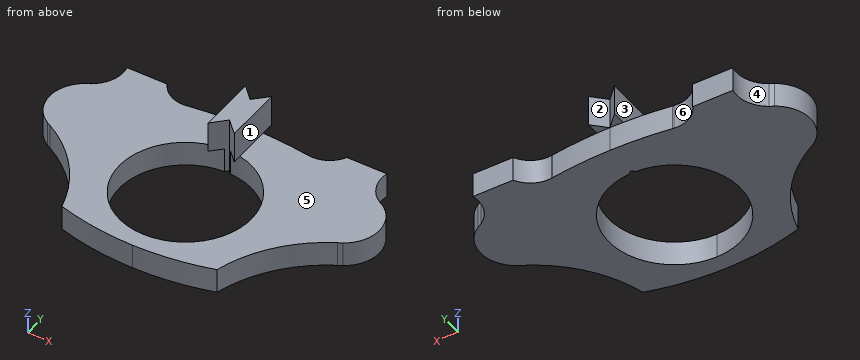
from build123d import *

# Parameters (mm, degrees)
F1_DEPTH = 8
F3_DEPTH = 10
F5_DEPTH = 25


with BuildPart() as f1:
    # F0 (on Top) → F1 (new body)
    with BuildSketch(Plane.XY):
        with BuildLine():
            Line((42.068422, 21.54067), (29.081911, 21.54067))
            ThreePointArc((29.081911, 21.54067), (25.256656, 17.577108), (19.841552, 16.567634))
            ThreePointArc((19.841552, 16.567634), (19.64703, 16.594249), (19.453131, 16.62508))
            ThreePointArc((19.453131, 16.62508), (9.752315, 17.686936), (0, 18.041513))
            ThreePointArc((0, 18.041513), (-9.752315, 17.686936), (-19.453131, 16.62508))
            ThreePointArc((-19.453131, 16.62508), (-19.64703, 16.594249), (-19.841552, 16.567634))
            ThreePointArc((-19.841552, 16.567634), (-25.256656, 17.577108), (-29.081911, 21.54067))
            Line((-29.081911, 21.54067), (-42.068422, 21.54067))
            ThreePointArc((-42.068422, 21.54067), (-42.606666, 15.286638), (-46.635796, 10.473247))
            ThreePointArc((-46.635796, 10.473247), (-47.308086, 10.078485), (-48.007976, 9.735025))
            ThreePointArc((-48.007976, 9.735025), (-53.385548, -0.095187), (-47.845987, -9.835033))
            ThreePointArc((-47.845987, -9.835033), (-47.228549, -10.153727), (-46.616208, -10.482108))
            ThreePointArc((-46.616208, -10.482108), (-33.037563, -21.996435), (-25.116532, -37.940607))
            ThreePointArc((-25.116532, -37.940607), (-12.686785, -40.637885), (0, -41.543091))
            ThreePointArc((0, -41.543091), (12.686785, -40.637885), (25.116532, -37.940607))
            ThreePointArc((25.116532, -37.940607), (33.037563, -21.996435), (46.616208, -10.482108))
            ThreePointArc((46.616208, -10.482108), (47.228549, -10.153727), (47.845987, -9.835033))
            ThreePointArc((47.845987, -9.835033), (53.385548, -0.095187), (48.007976, 9.735025))
            ThreePointArc((48.007976, 9.735025), (47.308086, 10.078485), (46.635796, 10.473247))
            ThreePointArc((46.635796, 10.473247), (42.606666, 15.286638), (42.068422, 21.54067))
        make_face()
        with BuildLine():
            ThreePointArc((0, 6.629357), (21.347405, -14.718047), (0, -36.065452))
            ThreePointArc((0, -36.065452), (-21.347405, -14.718047), (0, 6.629357))
        make_face(mode=Mode.SUBTRACT)
    extrude(amount=F1_DEPTH)

    # F2 (on face) → F3 (join)
    with BuildSketch(Plane.XY.offset(8)):
        Polygon((-4.242641, 3.38141), (0, 7.624051), (4.242641, 3.38141), (4.242641, 22.284153), (0, 18.041513), (-4.242641, 22.284153), align=None)
    extrude(amount=F3_DEPTH)

    # F4 (on face) → F5 (cut)
    with BuildSketch(Plane.XY.offset(18)):
        Polygon((4.242641, 3.38141), (0, 7.624051), (-4.242641, 3.38141), align=None)
    extrude(amount=-F5_DEPTH, mode=Mode.SUBTRACT)


solid = f1.part
Read the model definition and answer for the solid it produces. Units are mm, in the model's axes. Face numbers are marked on the shaded views. A direction names the side the tool comes from. Give positions to 0.01 mm unless a question says otherwise; leave off trailing zeros. Write each loop counter-clockwise with the first axis right and the second up, starting at its lowest first coordinate (ties: lowest second). Pieces come first, ordered by that corner, then holes. Notation, with made-up numbers: M 67.5,12 L 80.5,12 A35 cw 80.5,50 Z; hole C -37,79.5 d1. An arc over 180 degrees is marked long. One line per item, written item: value. Start each with the question number.
(1) A tool of negligible diameter and unlimited length cuts with its end or side. For the marked faces 1, 2 and 3, from which of +Z, -Z, +X, -X, +Y, -Y can it reach the whole face along a straight path? Write none if from no direction.
(2) Find section B-B (x = 12). Determine the outline of the cut face in (y, z).
(3) Find section D-D (z = 16.75). Determine the outline of the cut face in (x, y).
(4) Flat-ended cylindrical pins translate along their axes: pin 1 Ø8 at (y, z) = (-25, 3.5) entering from +X; pin 2 Ø2 at (x, y) = (13, 10.5) entering from +Z; pin 3 Ø2.5 at (x, y) = (2, 4.5) entering from -Z. Find the tip coordinate at first contact, or state that the pin passes through.
(5) Find section C-C (y = -30). Determine the outline of the cut face in (x, z).
(6) Find section A-A (z = 5.5). Determine the outline of the cut face in (x, y).
(7) Find the intervals of material crossed by line 1 (X direction, y = -2, z = 1.5); line 2 (X direction, y = -8, z = 6); line 3 (Y direction, x = -16, z = 2.5), in increasing order.
(8) Determine the mould class of the marked faces 4, 5 and 6 for opening direction Y: pulls with the +Y half, pulls with the -Y half, needs draft (parallel to the pull), parting line crosses it, or undercut.
Results below:
1. face 1: +Z, +X, +Y, -Y
1. face 2: +Z, -Z, +Y
1. face 3: +Z, -X, +Y, -Y
2. outline: M -40.73,0 L -32.37,0 L -32.37,8 L -40.73,8 Z; M 2.94,0 L 17.5,0 L 17.5,8 L 2.94,8 Z
3. outline: M -4.24,3.38 L 0,7.62 L 4.24,3.38 L 4.24,22.28 L 0,18.04 L -4.24,22.28 Z
4. pin 1: stops at x = 33.84
4. pin 2: stops at z = 8
4. pin 3: stops at z = 8
5. outline: M -28.05,0 L -14.91,0 L -14.91,8 L -28.05,8 Z; M 14.91,0 L 28.05,0 L 28.05,8 L 14.91,8 Z
6. outline: M -48.01,9.74 A11.5 ccw -47.85,-9.84 A44.11 cw -46.62,-10.48 A44.11 cw -25.12,-37.94 A89.36 ccw 0,-41.54 A89.36 ccw 25.12,-37.94 A44.11 cw 46.62,-10.48 A44.11 cw 47.85,-9.84 A11.5 ccw 48.01,9.74 A10.43 cw 46.64,10.47 A10.43 cw 42.07,21.54 L 29.08,21.54 A9.04 cw 19.84,16.57 A9.04 cw 19.45,16.63 A134.29 ccw 0,18.04 A134.29 ccw -19.45,16.63 A9.04 cw -19.84,16.57 A9.04 cw -29.08,21.54 L -42.07,21.54 A10.43 cw -46.64,10.47 A10.43 cw Z; hole M -1.02,6.61 A21.35 ccw long 1.02,6.61 L 0,7.62 Z
7. line 1: x = -53.21 to -17.15, 17.15 to 53.21
7. line 2: x = -50.15 to -20.26, 20.26 to 50.15
7. line 3: y = -40.1 to -28.85, -0.59 to 17.08
8. face 4: undercut
8. face 5: needs draft
8. face 6: pulls with the +Y half
